```python
from build123d import *

# Parameters (mm, degrees)
SKETCH1_R               = 12.5
BOSS_EXTRUDE1_DEPTH     = 14
FILLET2_R               = 1
SKETCH6_R               = 1
CUT_EXTRUDE2_DEPTH      = 5
SKETCH7_R               = 4.25
BOSS_EXTRUDE5_DEPTH     = 3
FILLET4_R               = 0.5
SKETCH8_R               = 2
BOSS_EXTRUDE6_DEPTH     = 12
CUT_EXTRUDE3_DEPTH      = 1
CUT_EXTRUDE3_DEPTH_BACK = 9
FILLET5_R               = 2


with BuildPart() as part:
    # Sketch1 → Boss-Extrude1 (new body)
    with BuildSketch(Plane.XY):
        Circle(SKETCH1_R)
    extrude(amount=BOSS_EXTRUDE1_DEPTH)

    # Fillet2
    fillet2_edges = [part.edges().sort_by_distance(p)[0] for p in [
        (-12.5, 0, 0),
    ]]
    fillet(fillet2_edges, radius=FILLET2_R)

    # Sketch6 → Cut-Extrude2 (cut)
    with BuildSketch(Plane(origin=(0, 0, 0), x_dir=(-1, 0, 0), z_dir=(0, 0, -1))):
        with Locations((-9.5, 0)):
            Circle(SKETCH6_R)
        with Locations((9.5, 0)):
            Circle(SKETCH6_R)
    extrude(amount=-CUT_EXTRUDE2_DEPTH, mode=Mode.SUBTRACT)

    # Sketch7 → Boss-Extrude5 (add)
    with BuildSketch(Plane(origin=(0, 0, 0), x_dir=(-1, 0, 0), z_dir=(0, 0, -1))):
        with Locations((0, -3)):
            Circle(SKETCH7_R)
    extrude(amount=BOSS_EXTRUDE5_DEPTH)

    # Fillet4
    fillet4_edges = [part.edges().sort_by_distance(p)[0] for p in [
        (4.25, -3, -3),
    ]]
    fillet(fillet4_edges, radius=FILLET4_R)

    # Sketch8 → Boss-Extrude6 (add)
    with BuildSketch(Plane(origin=(0, 0, -3), x_dir=(-1, 0, 0), z_dir=(0, 0, -1))):
        with Locations((0, -3)):
            Circle(SKETCH8_R)
    extrude(amount=BOSS_EXTRUDE6_DEPTH)

    # Sketch9 → Cut-Extrude3 (cut, two sides)
    with BuildSketch(Plane(origin=(0, 0, -15), x_dir=(-1, 0, 0), z_dir=(0, 0, -1))) as cut_extrude3_sk:
        Polygon((-53.075925999, -8.559326208), (-1.919066235, -2.436808394), (1.731963356, -1.999848545), (52.88882312, 4.122669269), (40.643787491, 106.436388797), (-65.320961628, 93.754393319), align=None)
    extrude(amount=CUT_EXTRUDE3_DEPTH, mode=Mode.SUBTRACT)
    extrude(cut_extrude3_sk.sketch, amount=-CUT_EXTRUDE3_DEPTH_BACK, mode=Mode.SUBTRACT)

    # Fillet5
    fillet5_edges = [part.edges().sort_by_distance(p)[0] for p in [
        (-12.5, 0, 14),
    ]]
    fillet(fillet5_edges, radius=FILLET5_R)


solid = part.part
```
For this review, take the finished solid that the model builds, in its own axes (mm). A direction names the side the tool comes from. Round coordinates to 2 decimals unless told otherwise and drop trailing zeros. Write each loop counter-clockwise with the first axis right and the second up, starting at its lowest first coordinate (ties: lowest second). Pieces come first, ordered by that corner, then holes.
1) For line 1 along X through (y, z) = (-0.75, 4); line 2 along Z through (x, y) = (-4, -6); line 3 along X through (y, z) = (-0.25, 1.25), list the stretches that pass through material, from the lowest coordinate up.
Answer below:
line 1: x = -12.48 to -10.16, -8.84 to 8.84, 10.16 to 12.48
line 2: z = 0 to 14
line 3: x = -12.5 to -10.47, -8.53 to 8.53, 10.47 to 12.5
2) Take a section at B-B on x = 0. Give the boundary of the cut face in (y, z).
Answer below:
outline: (-12.5, 1) arc R1 ccw to (-11.5, 0) - (-7.25, 0) - (-7.25, -2.5) arc R0.5 ccw to (-6.75, -3) - (-5, -3) - (-5, -15) - (-2.21, -15) - (-2.21, -6) - (-1, -6) - (-1, -3) - (0.75, -3) arc R0.5 ccw to (1.25, -2.5) - (1.25, 0) - (11.5, 0) arc R1 ccw to (12.5, 1) - (12.5, 12) arc R2 ccw to (10.5, 14) - (-10.5, 14) arc R2 ccw to (-12.5, 12) - close
3) Mouldability with a two-part tool opening along X and no side actions: class faces 4 (the face through (0, 3, 0)), 5 (the face through (0.12, -2.22, -10.56)), 6 (the face through (10.3, -0.6, 2.5)) as +X half, -X half, draft (parallel to the pull), parting line (faces both ways), or undercut.
Answer below:
face 4: draft
face 5: +X half
face 6: undercut
4) Machinability: for faces 1 (the face through (0, -3, -15)), 2 (the face through (0, -5, -9)), 3 (the face through (0, -2, -6)), which of the approach directions +Z, -Z, +X, -X, +Y, -Y give a long, thin tool a straight path to every point of the face, cutting with its end or side? Answer none if there is none.
Answer below:
face 1: -Z, +X, -X, +Y, -Y
face 2: -Z
face 3: -Z, +X, +Y
5) Insertion check: pin 1 Ø1 at (x, y) = (10, 0.5) entering from -Z; pin 2 Ø1 at (x, z) = (-4.5, 8) entering from +Y; pin 3 Ø1 at (y, z) = (8, 0) entering from +X. Each pin has a flat end and moves straight along its axis. Give the tip position at first contact, or say it passes through.
Answer below:
pin 1: stops at z = 0
pin 2: stops at y = 11.84
pin 3: stops at x = 9.59
6) Take a section at C-C on z = -1.75. Give the boundary of the cut face in (x, y).
Answer below:
outline: circle Ø8.5 at (0, -3)
7) Take a section at A-A on z = -9.25. Give the boundary of the cut face in (x, y), then the cut area to 3 significant figures.
Answer below:
outline: (-1.73, -2) arc R2 ccw (long way) to (1.92, -2.44) - close
area: 9.35 mm2
